Geometry check sheet. Reference: the model listing, model coordinates, mm. Face numbers are marked on the shaded views. A direction names the side the tool comes from. Round coordinates to 2 decimals unless told otherwise and drop trailing zeros. Order: outer loops, then holes, each group sorted by start corner. A loop starts at its lowest first (then second) coordinate and runs counter-clockwise, first axis right, second up. Notation, with made-up numbers: (-5.5, 46) -> (46.5, 46) arc R33 ccw to (46.5, 81) -> close; hole circle Ø3 at (8.25, 32). An arc over 180 degrees is marked (long way). Use a Markdown table: item, result. Add a question column.
Item 1: Material ranges on probe 1 along Z at (x, y) = (11.5, 4) (3 decimals); probe 2 along X at (y, z) = (4, 4.5); probe 3 along X at (y, z) = (3.75, 1.5), recorded low to high. Write a range as [from, to].
Item 2: Sectioned sample at A-A, the plane y = 2.5. Record the cut outline in (x, z) (3 decimals), and give its area (3 significant figures).
Item 3: Set-up check for the marked faces 4 and 5: record each of +Z, -Z, +X, -X, +Y, -Y from which the full face is reachable in a straight line by a thin tool's end or side.
Item 4: Mould release check, pull along Z, two halves, no side actions. Record for the marked faces 1, 2 and 3: pulls with the +Z half, pulls with the -Z half, needs draft (parallel to the pull), parting line crosses it, or undercut.
Item 5: Gauge pin test, flat ends, axial feed: pin 1 Ø2 at (y, z) = (2.5, -1) entering from -X; pin 2 Ø1.5 at (x, z) = (5, -1) entering from -Y; pin 3 Ø2.5 at (y, z) = (5, -4.5) entering from +X; pin 4 Ø0.7 at (x, y) = (29, 5) entering from +Z. Record the tip position at first contact, or that the pin passes through.
Item 6: Sectioned sample at C-C, the plane x = 19. Record the cut outline in (y, z) (3 decimals), and give its area (3 significant figures).
Item 7: Sectioned sample at B-B, the plane z = 4. Record the cut outline in (x, y), and give its area (3 significant figures).
from build123d import *

# Parameters (mm, degrees)
BOSS_EXTRUDE1_DEPTH = 6.55
SHELL1_T            = -1


with BuildPart() as part:
    # Sketch1 → Boss-Extrude1 (new body)
    with BuildSketch(Plane(origin=(0, 0, 0), x_dir=(1, 0, 0), z_dir=(0, 1, 0))):
        Polygon((28.31, 6.615), (28.31, 2.85), (29.21, 2.85), (29.21, -2.85), (28.31, -2.85), (28.31, -6.615), (-28.31, -6.615), (-28.31, -2.2), (-27.41, -2.2), (-27.41, 2.2), (-28.31, 2.2), (-28.31, 6.615), align=None)
    extrude(amount=BOSS_EXTRUDE1_DEPTH)

    # Shell1
    shell1_openings = [part.faces().sort_by_distance(p)[0] for p in [
        (0.3, 6.55, 0),
    ]]
    offset(amount=SHELL1_T, openings=shell1_openings, kind=Kind.INTERSECTION)


solid = part.part
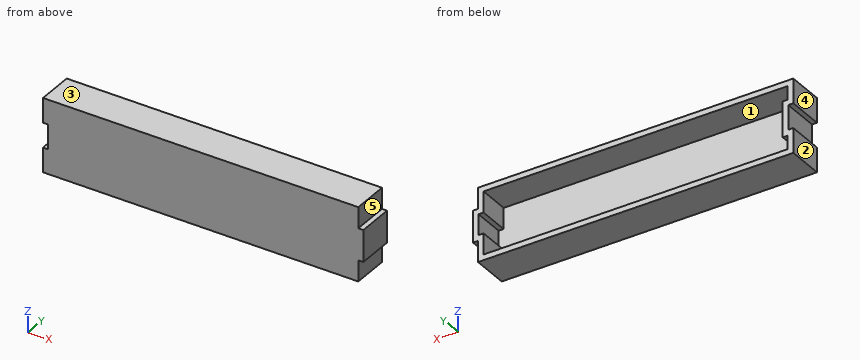
Found:
| question | item | result |
|---|---|---|
| 1 | probe 1 | z = [-6.615, -5.615], [5.615, 6.615] |
| 1 | probe 2 | x = [-28.31, -27.31], [27.31, 28.31] |
| 1 | probe 3 | x = [-27.41, -26.41], [28.21, 29.21] |
| 2 | outline | (-28.31, -6.615) -> (28.31, -6.615) -> (28.31, -2.85) -> (29.21, -2.85) -> (29.21, 2.85) -> (28.31, 2.85) -> (28.31, 6.615) -> (-28.31, 6.615) -> (-28.31, 2.2) -> (-27.41, 2.2) -> (-27.41, -2.2) -> (-28.31, -2.2) -> close; hole (-27.31, -5.615) -> (27.31, -5.615) -> (27.31, -1.85) -> (28.21, -1.85) -> (28.21, 1.85) -> (27.31, 1.85) -> (27.31, 5.615) -> (-27.31, 5.615) -> (-27.31, 3.2) -> (-26.41, 3.2) -> (-26.41, -3.2) -> (-27.31, -3.2) -> close |
| 2 | area | 139 mm2 |
| 3 | face 4 | +Z, -Z, -X, +Y, -Y |
| 3 | face 5 | +Z, +X, +Y, -Y |
| 4 | face 1 | undercut |
| 4 | face 2 | needs draft |
| 4 | face 3 | pulls with the +Z half |
| 5 | pin 1 | stops at x = -27.41 |
| 5 | pin 2 | stops at y = 0 |
| 5 | pin 3 | stops at x = 28.31 |
| 5 | pin 4 | stops at z = 2.85 |
| 6 | outline | (0, -6.615) -> (6.55, -6.615) -> (6.55, -5.615) -> (1, -5.615) -> (1, 5.615) -> (6.55, 5.615) -> (6.55, 6.615) -> (0, 6.615) -> close |
| 6 | area | 24.3 mm2 |
| 7 | outline | (-28.31, 0) -> (28.31, 0) -> (28.31, 6.55) -> (27.31, 6.55) -> (27.31, 1) -> (-27.31, 1) -> (-27.31, 6.55) -> (-28.31, 6.55) -> close |
| 7 | area | 67.7 mm2 |
